```python
from build123d import *

# Parameters (mm, degrees)
F1_DEPTH = 90
F2_R     = 3
F3_DEPTH = 68.7804190514
F4_R     = 3
F5_DEPTH = 68.7804190514


with BuildPart() as f1:
    # F0 (on Front) → F1 (new body)
    with BuildSketch(Plane.XZ):
        Polygon((-6.6202675138, 0), (0, 0), (57.053465335, 122.3515512499), (50.4331978212, 122.3515512499), align=None)
        Polygon((57.053465335, 122.3515512499), (0, 0), (6.6202675138, 0), (63.6737328488, 122.3515512499), align=None)
        Polygon((6.6202675138, 0), (0, 0), (0, -12), (63, -12), (63, 0), align=None)
        Polygon((0, -12), (0, 0), (-6.6202675138, 0), (-36, 0), (-36, -12), align=None)
    extrude(amount=F1_DEPTH)

    # F2 (on face) → F3 (cut, through all)
    with BuildSketch(Plane(origin=(-5.4378467222, 0, 2.5357095704), x_dir=(0, -1, 0), z_dir=(-0.906307787, 0, 0.4226182617))):
        with Locations((8, 122.2021540511)):
            Circle(F2_R)
        with Locations((82, 122.2021540511)):
            Circle(F2_R)
    extrude(amount=-F3_DEPTH, mode=Mode.SUBTRACT)

    # F4 (on face) → F5 (cut, through all)
    with BuildSketch(Plane(origin=(-5.4378467222, 0, 2.5357095704), x_dir=(0, -1, 0), z_dir=(-0.906307787, 0, 0.4226182617))):
        with Locations((12.5, 75.2021540511)):
            Circle(F4_R)
        with Locations((77.5, 75.2021540511)):
            Circle(F4_R)
    extrude(amount=-F5_DEPTH, mode=Mode.SUBTRACT)


solid = f1.part
```
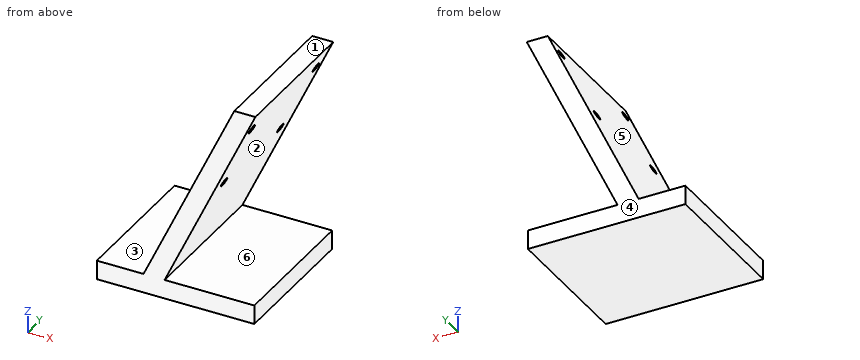
Design review of the part built by this model. Coordinates are the model's own, in mm. Face numbers are marked on the shaded views. A direction names the side the tool comes from. Coordinates: 2 decimals unless noted, no trailing zeros. Order: outer loops, then holes, each group sorted by start corner. A loop starts at its lowest first (then second) coordinate and runs counter-clockwise, first axis right, second up.
1) Mouldability with a two-part tool opening along Z and no side actions: class the marked faces 4, 5 and 6 as +Z half, -Z half, draft (parallel to the pull), parting line (faces both ways), or undercut.
2) For the marked faces 1, 2 and 3, list the 3-axis set-ups (+Z, -Z, +X, -X, +Y, -Y) from which the entire face can be reached by the end or side of a thin tool; tool diameter is ignored.
3) Wall thickness on line 1 along Z through (x, y) = (59, -72.5); line 2 along Z through (x, y) = (12.5, -56); line 3 along Z through (x, y) = (-20, -82.5): over which ranges is each line inside the solid? List them lowest first.
4) Take a section at B-B, the plane x = 52. State how many separate pieces and enclosed holes the cut face has, and give its area (3 significant figures).
5) Take a section at C-C, the plane z = 15.5. Give the boundary of the cut face in (x, y), and give its area (3 significant figures).
6) Take a section at D-D, the plane x = 0. Give the boundary of the cut face in (y, z), and give its area (3 significant figures).
7) Clearance check with flat-ended pins moving along their axes: pin 1 (4 mm diameter, centred on y = -13, z = 53, fed in from +X); pin 2 (6 mm diameter, centred on x = -22, y = -58.5, fed in from +Z); pin 3 (1.5 mm diameter, centred on x = -6.5, y = -64, fed in from +Z). State where each tip first meets the part, or that it passes through.
8) Take a section at A-A, the plane y = -44. Give the boundary of the cut face in (x, z).
Returned:
1. face 4: draft
1. face 5: +Z half
1. face 6: undercut
2. face 1: +Z, +X, -X, +Y, -Y
2. face 2: +X, +Y, -Y
2. face 3: +Z, -X, +Y, -Y
3. line 1: z = -12 to 0, 112.33 to 122.35
3. line 2: z = -12 to 0, 12.61 to 41
3. line 3: z = -12 to 0
4. separate pieces: 2
4. enclosed holes: 2
4. area: 3,270 mm2
5. outline: (0.61, -90) - (13.85, -90) - (13.85, 0) - (0.61, 0) - close
5. area: 1,190 mm2
6. outline: (-90, -12) - (0, -12) - (0, 14.2) - (-90, 14.2) - close
6. area: 2,360 mm2
7. pin 1: stops at x = 32.27
7. pin 2: stops at z = 0
7. pin 3: stops at z = 1.87
8. outline: (-36, -12) - (63, -12) - (63, 0) - (6.62, 0) - (63.67, 122.35) - (50.43, 122.35) - (-6.62, 0) - (-36, 0) - close
